```python
from build123d import *

# Parameters (mm, degrees)
BOSS_EXTRUDE1_START = -9
SKETCH2_W           = 10
SKETCH2_H           = 10
BOSS_EXTRUDE1_DEPTH = 5
BOSS_EXTRUDE2_START = -4
BOSS_EXTRUDE2_DEPTH = 4


with BuildPart() as part:
    # Sketch2 → Boss-Extrude1 (new body)
    with BuildSketch(Plane(origin=(0, 0, 0), x_dir=(0, 0, -1), z_dir=(1, 0, 0)).offset(BOSS_EXTRUDE1_START)):
        with BuildLine():
            Line((-20, 0), (-20, -200))
            Line((-20, -200), (20, -200))
            Line((20, -200), (20, 0))
            ThreePointArc((20, 0), (0, 20), (-20, 0))
        make_face()
        Rectangle(SKETCH2_W, SKETCH2_H, mode=Mode.SUBTRACT)
    extrude(amount=BOSS_EXTRUDE1_DEPTH)

    # Sketch2<6> → Boss-Extrude2 (add)
    with BuildSketch(Plane(origin=(0, 0, 0), x_dir=(0, 0, -1), z_dir=(1, 0, 0)).offset(BOSS_EXTRUDE2_START)):
        with BuildLine():
            Line((-20, 0), (-20, -200))
            Line((-20, -200), (20, -200))
            Line((20, -200), (20, 0))
            ThreePointArc((20, 0), (0, 20), (-20, 0))
        make_face()
        with BuildLine():
            Line((15, 0), (15, -195))
            Line((15, -195), (-15, -195))
            Line((-15, -195), (-15, 0))
            ThreePointArc((-15, 0), (0, 15), (15, 0))
        make_face(mode=Mode.SUBTRACT)
    extrude(amount=BOSS_EXTRUDE2_DEPTH)

    # Mirror1: part across plane


with BuildPart() as part_1:
    add(part.part)
    add(part.part.mirror(Plane(origin=(0, 0, 0), x_dir=(0, 0, 1), z_dir=(1, 0, 0))))


solid = part_1.part
```
Here's how the part is built. I have some questions about the finished solid (model axes, mm). A direction names the side the tool comes from. Give positions to 0.01 mm unless a question says otherwise; leave off trailing zeros. Loops run counter-clockwise (first coordinate to the right, second up) from the corner with the lowest first, then second, coordinate; pieces in that order, holes last. Notation, with made-up numbers: M 85,15.5 L 144,15.5 A28 cw 144,48.5 Z; hole C 5,-19.5 d11. An arc over 180 degrees is marked long. Use one line per item in the form item = value. Start each with the question number.
Q1. Will these pins go through, and if not, where does the flat tip stop? pin 1 Ø1.5 at (x, z) = (-6.5, -2) entering from +Y; pin 2 Ø4 at (x, z) = (1, -11) entering from +Y; pin 3 Ø2.5 at (x, z) = (-0.5, -3) entering from +Y.
Q2. I need wall thicknesses on line 1 along X through (y, z) = (-179.5, -10.5); line 2 along Z through (x, y) = (3.75, -61); line 3 along Y through (x, z) = (-7.75, -1). Which ranges of each line are inside material? Lowest first, please.
Q3. If we section it at C-C (x = -2): Write out the boundary of the cut face in (y, z), then the cut area to 3 significant figures.
Q4. Thinking about a two-plate mould opening in Z: for faces 4 (the flat face through (9, -88, 0)), 5 (the flat face through (0, -101, -20)), 6 (the flat face through (-4, -89, 0)), 7 (the flat face through (-7, -5, 0)), which applies, +Z half, -Z half, draft (parallel to the pull), parting line (faces both ways), or undercut?
Q5. If we section it at D-D (z = 17): Write out the boundary of the cut face in (x, y).
Q6. Which directions (+Z, -Z, +X, -X, +Y, -Y) give clear straight access to the entire face, cutting with the end or side of a thin tool? Please do faces 1 (the flat face through (-9, -88, 0)), 2 (the flat face through (4, -89, 0)), 3 (the flat face through (7, 0, 5)).
Q7. If we section it at B-B (y = -60.5): Write out the boundary of the cut face in (x, z), then the cut area to 3 significant figures.
Q8. If we section it at A-A (z = 0): Write out the boundary of the cut face in (x, y), then the cut area to 3 significant figures.
Taken from the geometry:
q1.pin_1 = 19.96
q1.pin_2 = 17.86
q1.pin_3 = 19.92
q2.line_1 = -9 to -4, 4 to 9
q2.line_2 = -20 to -15, 15 to 20
q2.line_3 = -200 to -5, 5 to 19.97
q3.outline = M -200,-20 L 0,-20 A20 ccw 0,20 L -200,20 Z; hole M -195,-15 L 0,-15 A15 ccw 0,15 L -195,15 Z
q3.area = 2,420 mm^2
q4.face_4 = draft
q4.face_5 = -Z half
q4.face_6 = undercut
q4.face_7 = undercut
q5.outline = M -9,-200 L 9,-200 L 9,10.54 L -9,10.54 Z
q6.face_1 = +Z, -Z, -X, +Y, -Y
q6.face_2 = none
q6.face_3 = +X, -X
q7.outline = M -9,-20 L 9,-20 L 9,20 L -9,20 Z; hole M -4,-15 L 4,-15 L 4,15 L -4,15 Z
q7.area = 480 mm^2
q8.outline = M -9,-200 L 9,-200 L 9,-5 L 4,-5 L 4,-195 L -4,-195 L -4,-5 L -9,-5 Z; M -9,5 L -4,5 L -4,15 L 4,15 L 4,5 L 9,5 L 9,20 L -9,20 Z
q8.area = 2,180 mm^2
